from build123d import *

# Parameters (mm, degrees)
SKETCH_3_R          = 178
EXTRUDE_3_DEPTH     = 3
SKETCH_4_R          = 10
SKETCH_4_R_2        = 5.3
CUT_EXTRUDE_1_DEPTH = 10
CUT_EXTRUDE_2_DEPTH = 10
SKETCH_6_R          = 2
SKETCH_6_W          = 120
SKETCH_6_H          = 5
CUT_EXTRUDE_3_DEPTH = 10


with BuildPart() as part:
    # 草图3 → 凸台-拉伸3 (new body)
    with BuildSketch(Plane(origin=(0, 0, 0), x_dir=(1, 0, 0), z_dir=(0, 1, 0))):
        Circle(SKETCH_3_R)
        with BuildLine():
            Line((-25, 33.75), (-25, -67.5))
            Line((-25, -67.5), (-116.913429511, -67.5))
            ThreePointArc((-116.913429511, -67.5), (-135, 0), (-116.913429511, 67.5))
            Line((-116.913429511, 67.5), (-25, 67.5))
            Line((-25, 67.5), (-25, 33.75))
        make_face(mode=Mode.SUBTRACT)
        with BuildLine():
            Line((25, 33.75), (25, 67.5))
            Line((25, 67.5), (116.913429511, 67.5))
            ThreePointArc((116.913429511, 67.5), (135, 0), (116.913429511, -67.5))
            Line((116.913429511, -67.5), (25, -67.5))
            Line((25, -67.5), (25, 33.75))
        make_face(mode=Mode.SUBTRACT)
    extrude(amount=EXTRUDE_3_DEPTH)

    # 草图4 → 切除-拉伸1 (cut)
    with BuildSketch(Plane(origin=(0, 3, 0), x_dir=(1, 0, 0), z_dir=(0, 1, 0))):
        with Locations((115.258405333, 115.258405333)):
            Circle(SKETCH_4_R)
        with Locations((115.258405333, -115.258405333)):
            Circle(SKETCH_4_R)
        with Locations((-115.258405333, -115.258405333)):
            Circle(SKETCH_4_R)
        with Locations((-115.258405333, 115.258405333)):
            Circle(SKETCH_4_R)
        with Locations((-90.216925784, -106.480381752)):
            Circle(SKETCH_4_R_2)
        with Locations((-106.480381752, -90.216925784)):
            Circle(SKETCH_4_R_2)
        with Locations((-106.480381752, 90.216925784)):
            Circle(SKETCH_4_R_2)
        with Locations((-90.216925784, 106.480381752)):
            Circle(SKETCH_4_R_2)
        with Locations((90.216925784, 106.480381752)):
            Circle(SKETCH_4_R_2)
        with Locations((106.480381752, 90.216925784)):
            Circle(SKETCH_4_R_2)
        with Locations((106.480381752, -90.216925784)):
            Circle(SKETCH_4_R_2)
        with Locations((90.216925784, -106.480381752)):
            Circle(SKETCH_4_R_2)
    extrude(amount=-CUT_EXTRUDE_1_DEPTH, mode=Mode.SUBTRACT)

    # 草图5 → 切除-拉伸2 (cut)
    with BuildSketch(Plane(origin=(0, 3, 0), x_dir=(1, 0, 0), z_dir=(0, 1, 0))):
        with BuildLine():
            Line((95.833188406, 150), (0, 150))
            Line((0, 150), (-95.833188406, 150))
            ThreePointArc((-95.833188406, 150), (0, 178), (95.833188406, 150))
        make_face()
        with BuildLine():
            Line((150, 95.833188406), (150, 0))
            Line((150, 0), (150, -95.833188406))
            ThreePointArc((150, -95.833188406), (178, 0), (150, 95.833188406))
        make_face()
        with BuildLine():
            Line((95.833188406, -150), (0, -150))
            Line((0, -150), (-95.833188406, -150))
            ThreePointArc((-95.833188406, -150), (0, -178), (95.833188406, -150))
        make_face()
        with BuildLine():
            Line((-150, 0), (-150, -95.833188406))
            ThreePointArc((-150, -95.833188406), (-178, 0), (-150, 95.833188406))
            Line((-150, 95.833188406), (-150, 0))
        make_face()
    extrude(amount=-CUT_EXTRUDE_2_DEPTH, mode=Mode.SUBTRACT)

    # 草图6 → 切除-拉伸3 (cut)
    with BuildSketch(Plane(origin=(0, 3, 0), x_dir=(1, 0, 0), z_dir=(0, 1, 0))):
        with Locations((35, -78)):
            Circle(SKETCH_6_R)
        with Locations((-35, -78)):
            Circle(SKETCH_6_R)
        with Locations((-35, 78)):
            Circle(SKETCH_6_R)
        with Locations((35, 78)):
            Circle(SKETCH_6_R)
        with Locations((0, -87.5)):
            Rectangle(SKETCH_6_W, SKETCH_6_H)
        with Locations((0, 87.5)):
            Rectangle(SKETCH_6_W, SKETCH_6_H)
    extrude(amount=-CUT_EXTRUDE_3_DEPTH, mode=Mode.SUBTRACT)


solid = part.part
Source: CAD feature listing. Evaluate the final solid. Frame: model axes, mm. A direction names the side the tool comes from. Round coordinates to 2 decimals unless told otherwise and drop trailing zeros. Loops run counter-clockwise (first coordinate to the right, second up) from the corner with the lowest first, then second, coordinate; pieces in that order, holes last. Notation, with made-up numbers: (-37, 84.25) - (-6, 84.25) arc R33 cw to (-6, 115.25) - close; hole circle Ø7 at (-14, 53.25). An arc over 180 degrees is marked (long way). Write item = value, one per line. Start each with the question number.
(1) Section query C-C, the plane z = 55. Output: boundary loops of the cut face in (x, y), plus the area to 3 significant figures.
(2) Section query B-B, the plane x = 72. Output: boundary loops of the cut face in (y, z), plus the area to 3 significant figures.
(3) Ray query, line 1 along Z through (x, y) = (-116, 0.6); line 2 along Z through (x, y) = (35, 2.4); line 3 along X through (y, z) = (2.35, -78). Return the intervals inside material, ascending. Write a range as from..to.
(4) Pull-direction query (Z, two-part tool) for faces 3 (the face through (-125.48, 1.48, -126.25)), 4 (the face through (107.323, 1.521, -109.174)), 5 (the face through (-2, 0, -2)), 6 (the face through (-126.25, 1.48, 125.48)); classes: +Z half, -Z half, draft (parallel to the pull), parting line (faces both ways), or undercut.
(5) Section query A-A, the plane x = -21. Output: boundary loops of the cut face in (y, z).
(6) Section query D-D, the plane y = 0.6. State how many separate pieces and enclosed holes the cut face has, plus the area to 3 significant figures.
(7) Set-up query: faces 1 (the face through (-2, 3, -2)), 2 (the face through (134.996, 1.479, -0.99)). Return all of +Z, -Z, +X, -X, +Y, -Y with unobstructed straight access to the full face (end or side cutting, diameter ignored); none if empty.
Conclusion:
q1.outline = (-150, 0) - (-123.29, 0) - (-123.29, 3) - (-150, 3) - close; (-25, 0) - (25, 0) - (25, 3) - (-25, 3) - close; (123.29, 0) - (150, 0) - (150, 3) - (123.29, 3) - close
q1.area = 310 mm2
q2.outline = (0, -150) - (3, -150) - (3, -67.5) - (0, -67.5) - close; (0, 67.5) - (3, 67.5) - (3, 150) - (0, 150) - close
q2.area = 495 mm2
q3.line_1 = -135.01..-125.23, -105.29..-67.5, 67.5..105.29, 125.23..135.01
q3.line_2 = -150..-90, -85..-80, -76..-67.5, 67.5..76, 80..85, 90..150
q3.line_3 = -150..-37, -33..33, 37..150
q4.face_3 = -Z half
q4.face_4 = undercut
q4.face_5 = draft
q4.face_6 = +Z half
q5.outline = (0, -150) - (3, -150) - (3, -90) - (0, -90) - close; (0, -85) - (3, -85) - (3, 85) - (0, 85) - close; (0, 90) - (3, 90) - (3, 150) - (0, 150) - close
q6.separate_pieces = 1
q6.enclosed_holes = 20
q6.area = 53,700 mm2
q7.face_1 = +Z, -Z, +X, -X, +Y
q7.face_2 = +Y, -Y
